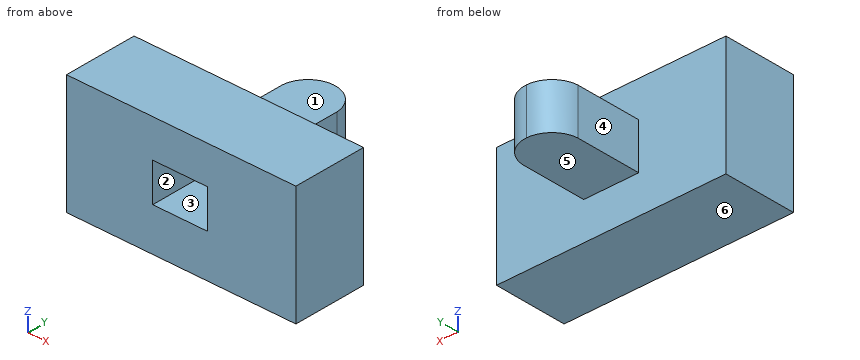
from build123d import *

# Parameters (mm, degrees)
SKETCH3_W           = 25
SKETCH3_H           = 13
BOSS_EXTRUDE1_DEPTH = 8
SKETCH4_W           = 6
SKETCH4_H           = 4.2
CUT_EXTRUDE1_DEPTH  = 7
SKETCH5_W           = 6
SKETCH5_H           = 5
BOSS_EXTRUDE2_DEPTH = 10
CUT_EXTRUDE2_DEPTH  = 10


with BuildPart() as part:
    # Sketch3 → Boss-Extrude1 (new body)
    with BuildSketch(Plane(origin=(0, 0, 0), x_dir=(1, 0, 0), z_dir=(0, 1, 0))):
        with Locations((6.675257732, -1.809278351)):
            Rectangle(SKETCH3_W, SKETCH3_H)
    extrude(amount=BOSS_EXTRUDE1_DEPTH)

    # Sketch4 → Cut-Extrude1 (cut)
    with BuildSketch(Plane.XZ):
        with Locations((6.568666205, 2.102026057)):
            Rectangle(SKETCH4_W, SKETCH4_H)
    extrude(amount=-CUT_EXTRUDE1_DEPTH, mode=Mode.SUBTRACT)

    # Sketch5 → Boss-Extrude2 (add)
    with BuildSketch(Plane(origin=(0, 8, 0), x_dir=(1, 0, 0), z_dir=(0, 1, 0))):
        with Locations((6.675257732, -1.902518117)):
            Rectangle(SKETCH5_W, SKETCH5_H)
    extrude(amount=BOSS_EXTRUDE2_DEPTH)

    # Sketch6 → Cut-Extrude2 (cut)
    with BuildSketch(Plane(origin=(0, 0, -0.597481883), x_dir=(-1, 0, 0), z_dir=(0, 0, -1))):
        with BuildLine():
            Line((-3.675257732, 18), (-6.675257732, 18))
            ThreePointArc((-6.675257732, 18), (-4.610198245, 17.177859086), (-3.675257732, 15.161358998))
            Line((-3.675257732, 15.161358998), (-3.675257732, 18))
        make_face()
        with BuildLine():
            Line((-9.675257732, 18), (-9.675257732, 15.161358998))
            ThreePointArc((-9.675257732, 15.161358998), (-8.740317219, 17.177859086), (-6.675257732, 18))
            Line((-6.675257732, 18), (-9.675257732, 18))
        make_face()
    extrude(amount=-CUT_EXTRUDE2_DEPTH, mode=Mode.SUBTRACT)


solid = part.part
Input: part model. Units: mm. Frame: model coordinates. Face numbers are marked on the shaded views. A direction names the side the tool comes from. Give positions to 0.01 mm unless a question says otherwise; leave off trailing zeros. Order: outer loops, then holes, each group sorted by start corner. A loop starts at its lowest first (then second) coordinate and runs counter-clockwise, first axis right, second up.
Q1. Set-up query: the marked faces 5 and 6. Return all of +Z, -Z, +X, -X, +Y, -Y with unobstructed straight access to the full face (end or side cutting, diameter ignored); none if empty.
Checked values:
face 5: -Z, +X, -X, +Y
face 6: -Z, +X, -X, +Y, -Y
Q2. Section A-A on y = 2.25. Output: boundary loops of the cut face in (x, z).
Checked values:
outline: (-5.82, -4.69) - (19.18, -4.69) - (19.18, 8.31) - (-5.82, 8.31) - close; hole (3.57, 0) - (9.57, 0) - (9.57, 4.2) - (3.57, 4.2) - close
Q3. Contact query for flat-ended pins moving along their axis: pin 1 Ø4 at (y, z) = (12, -0.5) entering from -X; pin 2 Ø3 at (x, z) = (-2, 4) entering from +Y; pin 3 Ø1.8 at (x, y) = (8, 13) entering from +Z; pin 4 Ø6 at (y, z) = (9, 1.5) entering from -X. Output: stop coordinate, or through.
Checked values:
pin 1: stops at x = 3.68
pin 2: stops at y = 8
pin 3: stops at z = 4.4
pin 4: stops at x = -5.82
Q4. Draft query along Z for the marked faces 1, 2, 3 and 4. Return one class per face: +Z half, -Z half, draft (parallel to the pull), parting line (faces both ways), or undercut.
Checked values:
face 1: +Z half
face 2: undercut
face 3: undercut
face 4: draft
Q5. Section C-C on x = 4.25. Output: boundary loops of the cut face in (y, z).
Checked values:
outline: (0, -4.69) - (8, -4.69) - (8, -0.6) - (16.77, -0.6) - (16.77, 4.4) - (8, 4.4) - (8, 8.31) - (0, 8.31) - (0, 4.2) - (7, 4.2) - (7, 0) - (0, 0) - close
Q6. Section D-D on y = 11. Output: boundary loops of the cut face in (x, z).
Checked values:
outline: (3.68, -0.6) - (9.68, -0.6) - (9.68, 4.4) - (3.68, 4.4) - close
Q7. Ray query, probe 1 along X at (y, z) = (6.75, 4); probe 2 along Z at (x, y) = (6.75, 3); probe 3 along Y at (x, z) = (16, 2.75). Return the intervals inside material, ascending.
Checked values:
probe 1: x = -5.82 to 3.57, 9.57 to 19.18
probe 2: z = -4.69 to 0, 4.2 to 8.31
probe 3: y = 0 to 8
Q8. Section B-B on z = 2. Output: boundary loops of the cut face in (x, y).
Checked values:
outline: (-5.82, 0) - (3.57, 0) - (3.57, 7) - (9.57, 7) - (9.57, 0) - (19.18, 0) - (19.18, 8) - (9.68, 8) - (9.68, 15.16) arc R3 ccw to (3.68, 15.16) - (3.68, 8) - (-5.82, 8) - close
